from build123d import *

# Parameters (mm, degrees)
EXTRUDE_1_DEPTH     = 40
SKETCH_2_R          = 18
EXTRUDE_2_DEPTH     = 8
EXTRUDE_START       = -8
SKETCH_3_R          = 18
EXTRUDE_3_DEPTH     = 8
SKETCH_4_R          = 25.25
CUT_EXTRUDE_1_DEPTH = 30
SKETCH_5_R          = 25.25
CUT_EXTRUDE_2_DEPTH = 30
SKETCH_6_R          = 10
CUT_EXTRUDE_3_DEPTH = 10
SKETCH_7_R          = 7.5
CUT_EXTRUDE_4_DEPTH = 8
SKETCH_8_R          = 12
CUT_EXTRUDE_5_DEPTH = 40
SKETCH_9_R          = 8
CUT_EXTRUDE_6_DEPTH = 40
SKETCH_10_R         = 3.4
CUT_EXTRUDE_7_DEPTH = 20
SKETCH_11_R         = 3
CUT_EXTRUDE_8_DEPTH = 12


with BuildPart() as part:
    # 草图1 → 凸台-拉伸1 (new body)
    with BuildSketch(Plane.XY):
        with BuildLine():
            Line((-48, -45), (48, -45))
            ThreePointArc((48, -45), (56.485281374, -41.485281374), (60, -33))
            Line((60, -33), (60, 33))
            ThreePointArc((60, 33), (56.485281374, 41.485281374), (48, 45))
            Line((48, 45), (-48, 45))
            ThreePointArc((-48, 45), (-56.485281374, 41.485281374), (-60, 33))
            Line((-60, 33), (-60, -33))
            ThreePointArc((-60, -33), (-56.485281374, -41.485281374), (-48, -45))
        make_face()
    extrude(amount=EXTRUDE_1_DEPTH)

    # 草图2 → 凸台-拉伸2 (add)
    with BuildSketch(Plane(origin=(0, 45, 0), x_dir=(1, 0, 0), z_dir=(0, 1, 0))):
        with Locations(Location((0, -25, 0), (0, 0, 236.442690238))):
            Circle(SKETCH_2_R)
    extrude(amount=EXTRUDE_2_DEPTH)

    # 草图3 → 凸台-拉伸3 (add)
    with BuildSketch(Plane(origin=(0, -45, 0), x_dir=(1, 0, 0), z_dir=(0, 1, 0)).offset(EXTRUDE_START)):
        with Locations(Location((0, -25, 0), (0, 0, 236.442690238))):
            Circle(SKETCH_3_R)
    extrude(amount=EXTRUDE_3_DEPTH)

    # 草图4 → 切除-拉伸1 (cut)
    with BuildSketch(Plane.XY.offset(40)):
        with Locations((-21, 0)):
            Circle(SKETCH_4_R)
    extrude(amount=-CUT_EXTRUDE_1_DEPTH, mode=Mode.SUBTRACT)

    # 草图5 → 切除-拉伸2 (cut)
    with BuildSketch(Plane.XY.offset(40)):
        with Locations((21, 0)):
            Circle(SKETCH_5_R)
    extrude(amount=-CUT_EXTRUDE_2_DEPTH, mode=Mode.SUBTRACT)

    # 草图6 → 切除-拉伸3 (cut)
    with BuildSketch(Plane.XY.offset(10)):
        with Locations((-21, 0)):
            Circle(SKETCH_6_R)
    extrude(amount=-CUT_EXTRUDE_3_DEPTH, mode=Mode.SUBTRACT)

    # 草图7 → 切除-拉伸4 (cut)
    with BuildSketch(Plane.XY.offset(10)):
        with Locations((21, 0)):
            Circle(SKETCH_7_R)
    extrude(amount=-CUT_EXTRUDE_4_DEPTH, mode=Mode.SUBTRACT)

    # 草图8 → 切除-拉伸5 (cut)
    with BuildSketch(Plane(origin=(0, -53, 0), x_dir=(1, 0, 0), z_dir=(0, 1, 0))):
        with Locations(Location((0, -25, 0), (0, 0, 270))):
            Circle(SKETCH_8_R)
    extrude(amount=CUT_EXTRUDE_5_DEPTH, mode=Mode.SUBTRACT)

    # 草图9 → 切除-拉伸6 (cut)
    with BuildSketch(Plane(origin=(0, 53, 0), x_dir=(1, 0, 0), z_dir=(0, 1, 0))):
        with Locations(Location((0, -25, 0), (0, 0, 270))):
            Circle(SKETCH_9_R)
    extrude(amount=-CUT_EXTRUDE_6_DEPTH, mode=Mode.SUBTRACT)

    # 草图10 → 切除-拉伸7 (cut)
    with BuildSketch(Plane.XY.offset(40)):
        with Locations((-46, 32)):
            Circle(SKETCH_10_R)
        with Locations((46, 32)):
            Circle(SKETCH_10_R)
        with Locations((-46, -32)):
            Circle(SKETCH_10_R)
        with Locations((46, -32)):
            Circle(SKETCH_10_R)
    extrude(amount=-CUT_EXTRUDE_7_DEPTH, mode=Mode.SUBTRACT)

    # 草图11 → 切除-拉伸8 (cut)
    with BuildSketch(Plane.XY.offset(40)):
        with Locations((-30, 33)):
            Circle(SKETCH_11_R)
        with Locations((30, -33)):
            Circle(SKETCH_11_R)
    extrude(amount=-CUT_EXTRUDE_8_DEPTH, mode=Mode.SUBTRACT)


solid = part.part
Model file for the job. Use its own axes, mm. A direction names the side the tool comes from. Give positions to 0.01 mm unless a question says otherwise; leave off trailing zeros. Order: outer loops, then holes, each group sorted by start corner. A loop starts at its lowest first (then second) coordinate and runs counter-clockwise, first axis right, second up. Notation, with made-up numbers: (3, -22.75) -> (61, -22.75) arc R10 cw to (61, -3.75) -> close; hole circle Ø4 at (12, -27). An arc over 180 degrees is marked (long way). Use CSV: the item, a comma, the result in double quotes.
1. Band-saw the part on C-C, the plane z = 22.5. Give the cut face in (x, y).
Outcome:
outline,"(-60, -33) arc R12 ccw to (-48, -45) -> (-17.83, -45) -> (-17.83, -53) -> (-11.74, -53) -> (-11.74, -23.49) arc R25.25 cw (long way) to (-7.6, 21.4) -> (-7.6, 53) -> (-17.83, 53) -> (-17.83, 45) -> (-48, 45) arc R12 ccw to (-60, 33) -> close; (7.6, 21.4) arc R25.25 cw (long way) to (11.74, -23.49) -> (11.74, -53) -> (17.83, -53) -> (17.83, -45) -> (48, -45) arc R12 ccw to (60, -33) -> (60, 33) arc R12 ccw to (48, 45) -> (17.83, 45) -> (17.83, 53) -> (7.6, 53) -> close; hole circle Ø6.8 at (-46, -32); hole circle Ø6.8 at (-46, 32); hole circle Ø6.8 at (46, -32); hole circle Ø6.8 at (46, 32)"
2. Band-saw the part on B-B, the plane x = -21. Give the cut face in (y, z), then the cut area to 4 significant figures.
Outcome:
outline,"(-45, 0) -> (-10, 0) -> (-10, 10) -> (-25.25, 10) -> (-25.25, 40) -> (-45, 40) -> close; (10, 0) -> (45, 0) -> (45, 40) -> (25.25, 40) -> (25.25, 10) -> (10, 10) -> close"
area,"1,885 mm²"
3. 3-axis set-ups, long thin cutter, end or side, ignore diameter. For faces 1 (the cylindrical face through (0.53, -38.11, 13.01)), 2 (the flat face through (-7.4, 53, 29.4)), 3 (the flat face through (46, -32, 20)): which of +Z, -Z, +X, -X, +Y, -Y reach the whole face in a straight line?
Outcome:
face 1,"-Y"
face 2,"+Z, -Z, +X, -X, +Y"
face 3,"+Z"
4. Band-saw the part on D-D, the plane y = -19.5. Give the cut face in (x, z).
Outcome:
outline,"(-60, 0) -> (60, 0) -> (60, 40) -> (37.04, 40) -> (37.04, 10) -> (4.96, 10) -> (4.96, 14.07) arc R12 cw to (-4.96, 14.07) -> (-4.96, 10) -> (-37.04, 10) -> (-37.04, 40) -> (-60, 40) -> close; (-4.96, 35.93) arc R12 cw to (4.96, 35.93) -> (4.96, 40) -> (-4.96, 40) -> close"
5. Mould opens along X. For faces 4 (the cylindrical face through (0, 38, 17)), 5 (the cylindrical face through (-56.39, 41.58, 19.72)), 6 (the flat face through (0, 45, 41)) say: +X half, -X half, draft (parallel to the pull), parting line (faces both ways), or undercut.
Outcome:
face 4,"undercut"
face 5,"-X half"
face 6,"draft"
6. Drill centre lines: line 1 along Z through (x, y) = (0, 33.5); line 2 along Y through (x, z) = (-21, 17); line 3 along X through (y, z) = (30.5, 27). Where is each one in solid material? Low to high. Write a range as from..to.
Outcome:
line 1,"0..17, 33..40"
line 2,"-45..-25.25, 25.25..45"
line 3,"-60..-49.05, -42.95..-7.75, 7.75..42.95, 49.05..60"
7. Band-saw the part on A-A, the plane z = 5. Give the cut face in (x, y), then the cut area to 3 significant figures.
Outcome:
outline,"(-60, -33) arc R12 ccw to (-48, -45) -> (48, -45) arc R12 ccw to (60, -33) -> (60, 33) arc R12 ccw to (48, 45) -> (-48, 45) arc R12 ccw to (-60, 33) -> close; hole circle Ø20 at (-21, 0); hole circle Ø15 at (21, 0)"
area,"10,200 mm²"
8. Drop flat-ended pins along their axis: pin 1 (11 mm diameter, centred on x = 46, y = -32, fed in from +Z); pin 2 (2 mm diameter, centred on x = 47.5, y = -30.5, fed in from +Z); pin 3 (1.5 mm diameter, centred on x = -16.5, y = 8.5, fed in from +Z). Give the stop position or say it passes through.
Outcome:
pin 1,"z = 40"
pin 2,"z = 20"
pin 3,"z = 10"
